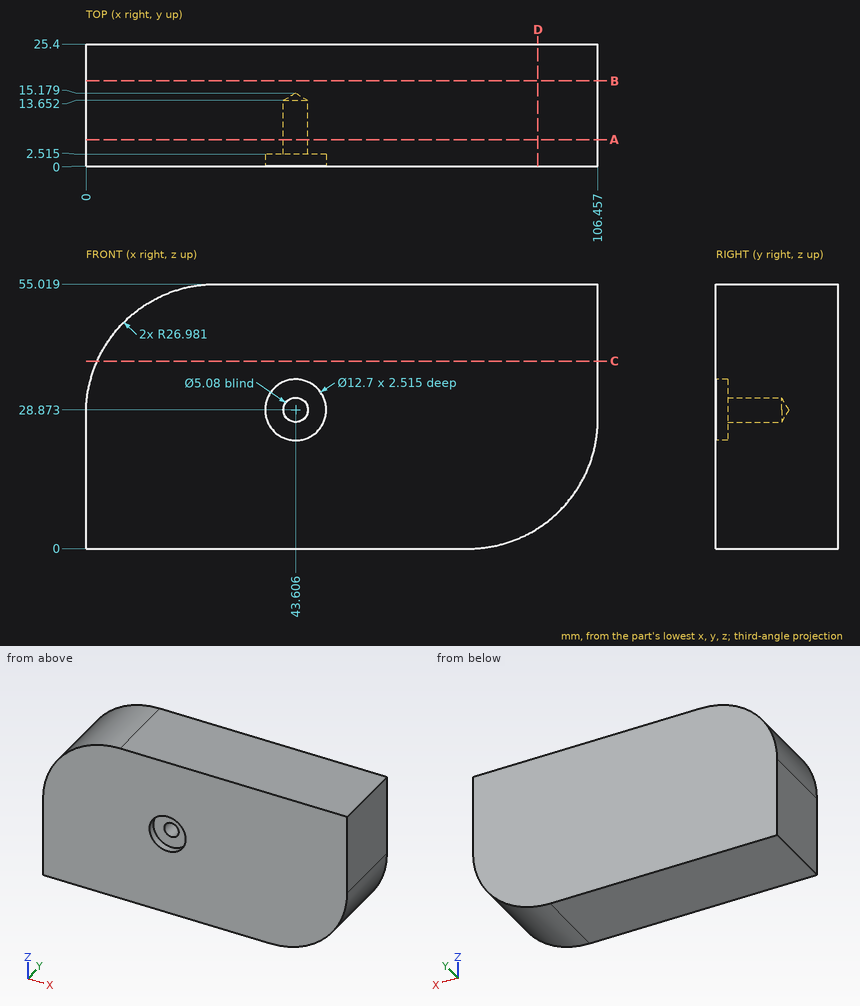
The drawing under review shows one solid part. Ordinate dimensions are in mm from its lowest x, y, z. Coordinates: 2 decimals unless noted, no trailing zeros. Write each loop counter-clockwise with the first axis right and the second up, starting at its lowest first coordinate (ties: lowest second). Pieces come first, ordered by that corner, then holes.
1) Add section D-D (x = 94). Write out the cut boundary in (y, z).
2) Add section A-A (y = 5.5). Write out the cut boundary in (x, z) (1 decimal).
3) To check wall thickness, follow L1, parallel to X at y = 6, z = 29.5 (1 decimal); L2, parallel to X at y = 19.25, z = 26.5; L3, parallel to Z at x = 42, y = 12 (1 decimal). State the ranges of each line that lie inside material, in increasing order.
4) Insertion check: pin 1 (1 mm diameter, centred on x = 42.5, z = 16.5, fed in from -Y); pin 2 (4.5 mm diameter, centred on x = 43.61, z = 28.87, fed in from -Y) (1 decimal); pin 3 (6.5 mm diameter, centred on x = 44, z = 29.5, fed in from -Y) (1 decimal); pin 4 (4 mm diameter, centred on y = 8, z = 48, fed in from -X). Each pin has a flat end and moves straight along its axis. Give the tip position at first contact, or say it passes through.
5) Add section C-C (z = 39). Write out the cut boundary in (x, y).
6) Add section B-B (y = 17.75). Write out the cut boundary in (x, z) (1 decimal).
Check result:
1. outline: (0, 4.24) - (25.4, 4.24) - (25.4, 55.02) - (0, 55.02) - close
2. outline: (0, 0) - (79.5, 0) arc R27 ccw to (106.5, 27) - (106.5, 55) - (27, 55) arc R27 ccw to (0, 28) - close; hole circle Ø5.1 at (43.6, 28.9)
3. L1: x = 0 to 41.1, 46.1 to 106.5
3. L2: x = 0 to 106.45
3. L3: z = 0 to 26.9, 30.8 to 55
4. pin 1: stops at y = 0
4. pin 2: stops at y = 13.8
4. pin 3: stops at y = 2.5
4. pin 4: stops at x = 6.85
5. outline: (2.33, 0) - (106.46, 0) - (106.46, 25.4) - (2.33, 25.4) - close
6. outline: (0, 0) - (79.5, 0) arc R27 ccw to (106.5, 27) - (106.5, 55) - (27, 55) arc R27 ccw to (0, 28) - close
